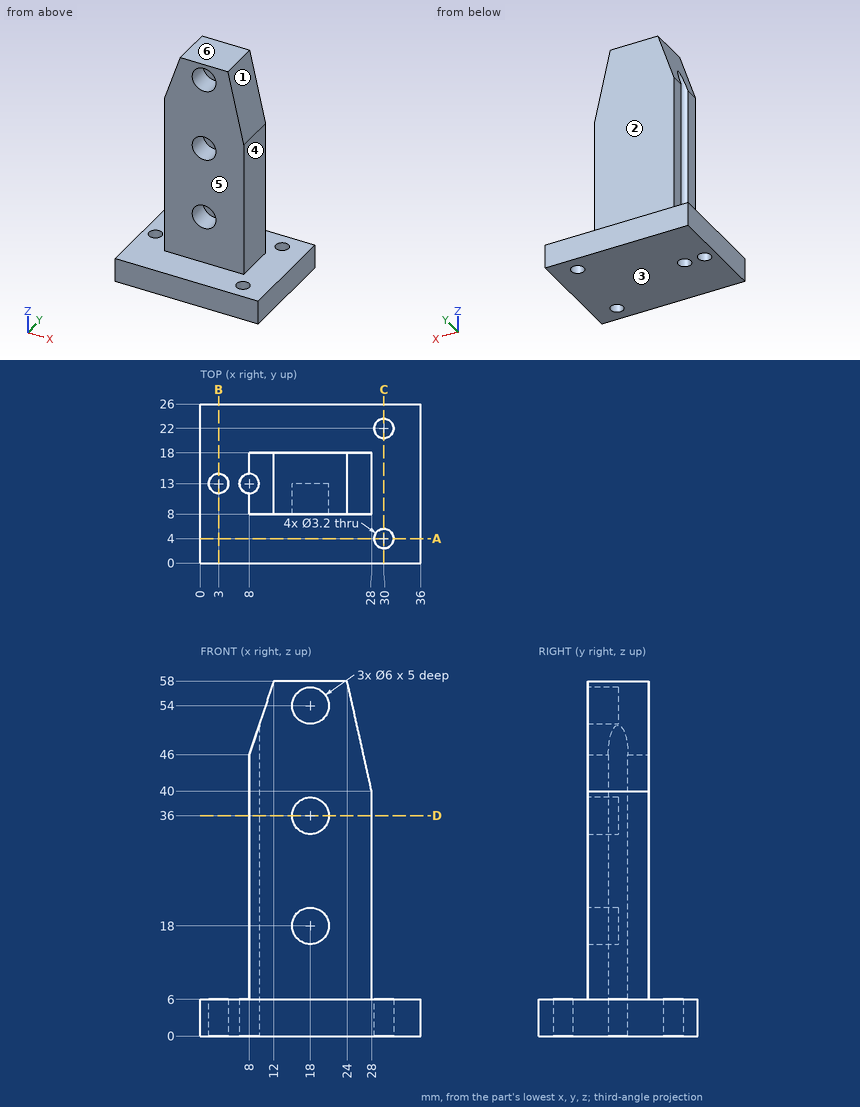
Geometry: see drawing. Coordinates: mm, zero at the bounding-box minimum. A direction names the side the tool comes from. Coordinates: 2 decimals unless noted, no trailing zeros. Loops run counter-clockwise (first coordinate to the right, second up) from the corner with the lowest first, then second, coordinate; pieces in that order, holes last. Notation, with made-up numbers: (24, 22.5) - (56, 22.5) arc R15 ccw to (56, 43.5) - close; hole circle Ø6 at (-18.5, 20.25). An arc over 180 degrees is marked (long way). Put each result on its own line as item: value. Start each with the question number.
Q1. Cut plane A-A, the plane y = 4. Return loops of the section in (x, z), and give its area (3 significant figures).
Q2. Cut plane D-D, the plane z = 36. Return loops of the section in (x, y).
Q3. Cut plane B-B, the plane x = 3. Return loops of the section in (y, z), and give its area (3 significant figures).
Q4. Set-up query: the marked faces 4, 5 and 6. Return all of +Z, -Z, +X, -X, +Y, -Y with unobstructed straight access to the full face (end or side cutting, diameter ignored); none if empty.
Q5. Pull-direction query (Z, two-part tool) for the marked faces 1, 2 and 3; classes: released by +Z, released by -Z, zero draft, split by the parting line, or undercut.
Q6. Line query: line 1 (Y direction, x = 30, z = 3); line 2 (X direction, y = 4, z = 4.3); line 3 (X direction, y = 10.1, z = 36). Output: solid intervals per line, ascending.
Q7. Pin query (flat end, axial travel): pin 1 Ø10 at (x, z) = (16, 25.5) entering from +Y; pin 2 Ø10 at (y, z) = (20, 24) entering from +X; pin 3 Ø2.5 at (y, z) = (10, 34.5) entering from -X; pin 4 Ø3 at (y, z) = (20, 14.5) entering from +X. Return the tip coordinate at first contact, or that it passes through.
Q8. Cut plane C-C, the plane x = 30. Return loops of the section in (y, z).
Filled sheet:
1. outline: (0, 0) - (28.4, 0) - (28.4, 6) - (0, 6) - close; (31.6, 0) - (36, 0) - (36, 6) - (31.6, 6) - close
1. area: 197 mm²
2. outline: (8, 8) - (15, 8) - (15, 13) - (21, 13) - (21, 8) - (28, 8) - (28, 18) - (8, 18) - (8, 14.6) arc R1.6 cw to (8, 11.4) - close
3. outline: (0, 0) - (11.4, 0) - (11.4, 6) - (0, 6) - close; (14.6, 0) - (26, 0) - (26, 6) - (14.6, 6) - close
3. area: 137 mm²
4. face 4: +Z, +X, +Y, -Y
4. face 5: +Z, +X, -X, -Y
4. face 6: +Z, +X, -X, +Y, -Y
5. face 1: released by +Z
5. face 2: zero draft
5. face 3: released by -Z
6. line 1: 0 to 2.4, 5.6 to 20.4, 23.6 to 26
6. line 2: 0 to 28.4, 31.6 to 36
6. line 3: 8 to 15, 21 to 28
7. pin 1: y = 18
7. pin 2: x = 28
7. pin 3: x = 8
7. pin 4: through
8. outline: (0, 0) - (2.4, 0) - (2.4, 6) - (0, 6) - close; (5.6, 0) - (20.4, 0) - (20.4, 6) - (5.6, 6) - close; (23.6, 0) - (26, 0) - (26, 6) - (23.6, 6) - close
